from build123d import *

# Parameters (mm, degrees)
SKETCH2_W           = 40
SKETCH2_H           = 30
SKETCH2_W_2         = 80
SKETCH2_H_2         = 50
SKETCH2_W_3         = 34.54
SKETCH2_H_3         = 5
BOSS_EXTRUDE5_DEPTH = 33
CUT_EXTRUDE1_DEPTH  = 25
SKETCH5_W           = 40
SKETCH5_H           = 40
CUT_EXTRUDE2_DEPTH  = 3
SKETCH6_W           = 41
SKETCH6_H           = 31
SKETCH6_W_2         = 40
SKETCH6_H_2         = 30
BOSS_EXTRUDE6_DEPTH = 30
SKETCH7_W           = 82
SKETCH7_H           = 52
SKETCH7_W_2         = 80
SKETCH7_H_2         = 50
CUT_EXTRUDE3_DEPTH  = 5
SKETCH8_R           = 2.5
BOSS_EXTRUDE7_DEPTH = 5
SKETCH10_W          = 7.223837829
SKETCH10_H          = 31
CUT_EXTRUDE6_DEPTH  = 41
SKETCH14_R          = 2
CUT_EXTRUDE9_DEPTH  = 20
SKETCH9_W           = 8.06
SKETCH9_H           = 3
CUT_EXTRUDE11_DEPTH = 5


with BuildPart() as part:
    # Sketch2 → Boss-Extrude5 (new body)
    with BuildSketch(Plane.XY):
        with BuildLine():
            ThreePointArc((-76.48364315, 74.732394366), (-90.625778773, 68.87452999), (-96.48364315, 54.732394366))
            Line((-96.48364315, 54.732394366), (-96.48364315, -35.267605634))
            ThreePointArc((-96.48364315, -35.267605634), (-90.625778773, -49.409741258), (-76.48364315, -55.267605634))
            Line((-76.48364315, -55.267605634), (63.51635685, -55.267605634))
            ThreePointArc((63.51635685, -55.267605634), (77.658492474, -49.409741258), (83.51635685, -35.267605634))
            Line((83.51635685, -35.267605634), (83.51635685, 54.732394366))
            ThreePointArc((83.51635685, 54.732394366), (77.658492474, 68.87452999), (63.51635685, 74.732394366))
            Line((63.51635685, 74.732394366), (-76.48364315, 74.732394366))
        make_face()
        with Locations((43.51635685, -10.267605634)):
            Rectangle(SKETCH2_W, SKETCH2_H, mode=Mode.SUBTRACT)
        with BuildLine():
            ThreePointArc((-86.48364315, -5), (-85.019177056, -1.464466094), (-81.48364315, 0))
            Line((-81.48364315, 0), (8.51635685, 0))
            ThreePointArc((8.51635685, 0), (12.051890756, -1.464466094), (13.51635685, -5))
            Line((13.51635685, -5), (13.51635685, -35))
            ThreePointArc((13.51635685, -35), (12.051890756, -38.535533906), (8.51635685, -40))
            Line((8.51635685, -40), (-81.48364315, -40))
            ThreePointArc((-81.48364315, -40), (-85.019177056, -38.535533906), (-86.48364315, -35))
            Line((-86.48364315, -35), (-86.48364315, -5))
        make_face(mode=Mode.SUBTRACT)
        with Locations((-36.48364315, 29.732394366)):
            Rectangle(SKETCH2_W_2, SKETCH2_H_2, mode=Mode.SUBTRACT)
        with Locations((43.51635685, 50.069459439)):
            Rectangle(SKETCH2_W_3, SKETCH2_H_3, mode=Mode.SUBTRACT)
        with Locations((43.51635685, 40.069459439)):
            Rectangle(SKETCH2_W_3, SKETCH2_H_3, mode=Mode.SUBTRACT)
    extrude(amount=BOSS_EXTRUDE5_DEPTH)

    # Sketch4 → Cut-Extrude1 (cut)
    with BuildSketch(Plane.XY.offset(33)):
        with BuildLine():
            Line((-81.48364315, 69.732394366), (68.51635685, 69.732394366))
            ThreePointArc((68.51635685, 69.732394366), (75.587424662, 66.803462178), (78.51635685, 59.732394366))
            Line((78.51635685, 59.732394366), (78.51635685, -40.267605634))
            ThreePointArc((78.51635685, -40.267605634), (75.587424662, -47.338673446), (68.51635685, -50.267605634))
            Line((68.51635685, -50.267605634), (-81.48364315, -50.267605634))
            ThreePointArc((-81.48364315, -50.267605634), (-88.554710961, -47.338673446), (-91.48364315, -40.267605634))
            Line((-91.48364315, -40.267605634), (-91.48364315, 59.732394366))
            ThreePointArc((-91.48364315, 59.732394366), (-88.554710961, 66.803462178), (-81.48364315, 69.732394366))
        make_face()
    extrude(amount=-CUT_EXTRUDE1_DEPTH, mode=Mode.SUBTRACT)

    # Sketch5 → Cut-Extrude2 (cut)
    with BuildSketch(Plane.XY.offset(8)):
        with Locations((43.51635685, 44.732394366)):
            Rectangle(SKETCH5_W, SKETCH5_H)
    extrude(amount=-CUT_EXTRUDE2_DEPTH, mode=Mode.SUBTRACT)

    # Sketch6 → Boss-Extrude6 (add)
    with BuildSketch(Plane.XY.offset(8)):
        with Locations((43.51635685, -10.267605634)):
            Rectangle(SKETCH6_W, SKETCH6_H)
        with Locations((43.51635685, -10.267605634)):
            Rectangle(SKETCH6_W_2, SKETCH6_H_2, mode=Mode.SUBTRACT)
    extrude(amount=BOSS_EXTRUDE6_DEPTH)

    # Sketch7 → Cut-Extrude3 (cut)
    with BuildSketch(Plane.XY.offset(8)):
        with Locations((-36.48364315, 29.732394366)):
            Rectangle(SKETCH7_W, SKETCH7_H)
        with Locations((-36.48364315, 29.732394366)):
            Rectangle(SKETCH7_W_2, SKETCH7_H_2, mode=Mode.SUBTRACT)
    extrude(amount=-CUT_EXTRUDE3_DEPTH, mode=Mode.SUBTRACT)

    # Sketch8 → Boss-Extrude7 (add)
    with BuildSketch(Plane.XY.offset(8)):
        with Locations((-77.48364315, 65.732394366)):
            Circle(SKETCH8_R)
        with Locations((17.51635685, 65.732394366)):
            Circle(SKETCH8_R)
        with Locations((-61.48364315, -43.947605634)):
            Circle(SKETCH8_R)
        with Locations((17.51635685, -43.447605634)):
            Circle(SKETCH8_R)
    extrude(amount=BOSS_EXTRUDE7_DEPTH)

    # Sketch10 → Cut-Extrude6 (cut)
    with BuildSketch(Plane.ZY.offset(-23.01635685)):
        with Locations((34.388081086, -10.267605634)):
            Rectangle(SKETCH10_W, SKETCH10_H)
    extrude(amount=-CUT_EXTRUDE6_DEPTH, mode=Mode.SUBTRACT)

    # Sketch14 → Cut-Extrude9 (cut)
    with BuildSketch(Plane.XY.offset(33)):
        with Locations((-93.98364315, 51.732394366)):
            Circle(SKETCH14_R)
        with Locations((81.01635685, 51.732394366)):
            Circle(SKETCH14_R)
        with Locations((81.01635685, -32.267605634)):
            Circle(SKETCH14_R)
        with Locations((-93.98364315, -32.267605634)):
            Circle(SKETCH14_R)
    extrude(amount=-CUT_EXTRUDE9_DEPTH, mode=Mode.SUBTRACT)

    # Sketch9 → Cut-Extrude11 (cut)
    with BuildSketch(Plane.ZY.offset(96.48364315)):
        with Locations((17.03, 6.418155037)):
            Rectangle(SKETCH9_W, SKETCH9_H)
    extrude(amount=-CUT_EXTRUDE11_DEPTH, mode=Mode.SUBTRACT)


solid = part.part
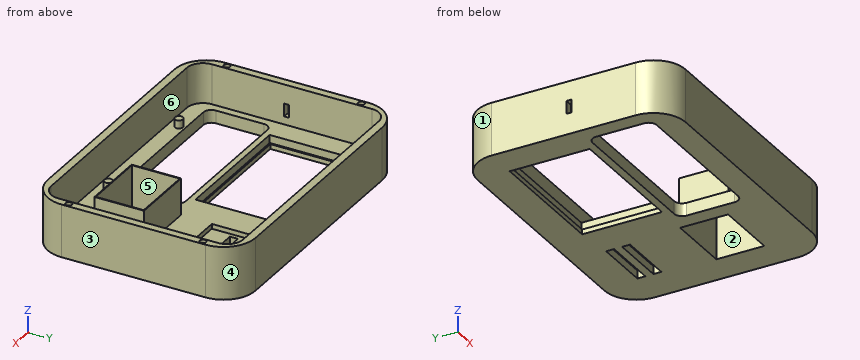
The listing builds one solid part. Answer for the finished solid, in the listing's coordinates (mm). Face numbers are marked on the shaded views. A direction names the side the tool comes from. Coordinates: 2 decimals unless noted, no trailing zeros. Order: outer loops, then holes, each group sorted by start corner. A loop starts at its lowest first (then second) coordinate and runs counter-clockwise, first axis right, second up. Notation, with made-up numbers: (-31, -27.75) -> (-16, -27.75) arc R32 ccw to (-16, 10.25) -> close; hole circle Ø7 at (47.25, 57). An arc over 180 degrees is marked (long way). Answer in a Markdown table with one row per item. Add a question column.
Item 1: Which of the six approach directions +Z, -Z, +X, -X, +Y, -Y give full straight-line access (tool end or side, diameter ignored) to the marked faces 4, 5 and 6?
Item 2: Find section A-A (y = 35.5). Write down the section's boundary in (x, z), then the cut area to 3 significant figures.
Item 3: Find the intervals of material crossed by L1, parallel to Y at x = 54.5, z = 13.5; L2, parallel to Y at x = -72.5, z = 2; L3, parallel to X at y = -12.5, z = 26.5, in increasing order. Write a range as from..to.
Item 4: Find section C-C (z = 19). State how many separate pieces and enclosed holes the cut face has, then the cut area to 3 significant figures.
Item 5: Find section D-D (x = -23.5). Write down the section's boundary in (y, z), then the cut area to 3 significant figures.
Item 6: Determine the mould class of the marked faces 1, 2 and 3 for opening direction Y: +Y half, -Y half, draft (parallel to the pull), parting line (faces both ways), or undercut.
Item 7: Each of these flat-tipped pins is pushed along its axis until it touches: P1, Ø3, axis at x = 7, y = 32, coming from the -Z side; P2, Ø1.5, axis at x = 18, y = 65.5, coming from the +Z side. Where does it stop, or does it pass through?
Item 8: Find section B-B (y = -8.5). Write down the section's boundary in (x, z).
Result set:
| question | item | result |
|---|---|---|
| 1 | face 4 | +Z, -Z, +X, +Y |
| 1 | face 5 | +Z, -Z |
| 1 | face 6 | +Z |
| 2 | outline | (-96.48, 0) -> (-76.48, 0) -> (-76.48, 3) -> (-77.48, 3) -> (-77.48, 8) -> (-91.48, 8) -> (-91.48, 33) -> (-96.48, 33) -> close; (3.52, 0) -> (83.52, 0) -> (83.52, 33) -> (78.52, 33) -> (78.52, 8) -> (63.52, 8) -> (63.52, 5) -> (23.52, 5) -> (23.52, 8) -> (4.52, 8) -> (4.52, 3) -> (3.52, 3) -> close |
| 2 | area | 920 mm² |
| 3 | L1 | y = -55.27..-50.27, -25.77..-25.27, 4.73..5.23, 69.73..74.73 |
| 3 | L2 | y = -55.27..-40, 0..4.73, 54.73..74.73 |
| 3 | L3 | x = -96.48..-91.48, 23.02..23.52, 63.52..64.02, 78.52..83.52 |
| 4 | separate pieces | 2 |
| 4 | enclosed holes | 5 |
| 4 | area | 2,750 mm² |
| 5 | outline | (-55.27, 0) -> (-40, 0) -> (-40, 8) -> (-50.27, 8) -> (-50.27, 33) -> (-55.27, 33) -> close; (0, 0) -> (4.73, 0) -> (4.73, 3) -> (3.73, 3) -> (3.73, 8) -> (0, 8) -> close; (54.73, 0) -> (74.73, 0) -> (74.73, 33) -> (69.73, 33) -> (69.73, 8) -> (55.73, 8) -> (55.73, 3) -> (54.73, 3) -> close |
| 5 | area | 560 mm² |
| 6 | face 1 | +Y half |
| 6 | face 2 | undercut |
| 6 | face 3 | draft |
| 7 | P1 | stops at z = 0 |
| 7 | P2 | stops at z = 13 |
| 8 | outline | (-96.48, 0) -> (-86.48, 0) -> (-86.48, 8) -> (-91.48, 8) -> (-91.48, 33) -> (-96.48, 33) -> close; (13.52, 0) -> (23.52, 0) -> (23.52, 30.78) -> (23.02, 30.78) -> (23.02, 8) -> (13.52, 8) -> close; (63.52, 0) -> (83.52, 0) -> (83.52, 33) -> (78.52, 33) -> (78.52, 8) -> (64.02, 8) -> (64.02, 30.78) -> (63.52, 30.78) -> close |
